```python
from build123d import *

# Parameters (mm, degrees)
F0_R     = 2
F0_R_2   = 2.2544770367
F1_DEPTH = 2


# Not quite as in the source:
# - ends of sketch curves that miss each other by under 0.0002 mm in the source are joined


with BuildPart() as f1:
    # F0 (on Top) → F1 (new body)
    with BuildSketch(Plane.XY):
        with BuildLine():
            ThreePointArc((-5.1683257468, -1.8810659147), (0, -5.5), (5.1683257468, -1.8810659147))
            Line((5.1683257468, -1.8810659147), (8.0301481547, -37.2918741238))
            ThreePointArc((8.0301481547, -37.2918741238), (9.2788304803, -38.3188106152), (10.2640215975, -37.0369352038))
            Line((10.2640215975, -37.0369352038), (3.1098692343, 51.4850906656))
            ThreePointArc((3.1098692343, 51.4850906656), (3.2758505583, 55.7142948477), (4.0791085727, 59.8698326439))
            Line((4.0791085727, 59.8698326439), (4.6310273864, 62.2435739623))
            ThreePointArc((4.6310273864, 62.2435739623), (6.6977396132, 71.4003991777), (3.5793046773, 80.2544440729))
            ThreePointArc((3.5793046773, 80.2544440729), (2.9779070013, 81.3790562482), (2.6805769718, 82.6192282376))
            Line((2.6805769718, 82.6192282376), (2.0130627379, 88.8089160456))
            ThreePointArc((2.0130627379, 88.8089160456), (1.9844093078, 88.9043745509), (1.9233044553, 88.9831117232))
            Line((1.9233044553, 88.9831117232), (0.9, 89.8927152157))
            Line((0.9, 89.8927152157), (0.9, 77.4665676321))
            ThreePointArc((0.9, 77.4665676321), (3.1034376701, 73.0014155649), (2.7328648238, 68.0359955106))
            ThreePointArc((2.7328648238, 68.0359955106), (1.8069828059, 67.0668885057), (0.5256445201, 66.6736988627))
            ThreePointArc((0.5256445201, 66.6736988627), (0.2620789214, 66.6755874914), (0, 66.7036058899))
            ThreePointArc((0, 66.7036058899), (-0.2620789214, 66.6755874914), (-0.5256445201, 66.6736988627))
            ThreePointArc((-0.5256445201, 66.6736988627), (-1.8069828059, 67.0668885057), (-2.7328648238, 68.0359955106))
            ThreePointArc((-2.7328648238, 68.0359955106), (-3.1034376701, 73.0014155649), (-0.9, 77.4665676321))
            Line((-0.9, 77.4665676321), (-0.9, 89.8927152157))
            Line((-0.9, 89.8927152157), (-1.9233044553, 88.9831117232))
            ThreePointArc((-1.9233044553, 88.9831117232), (-1.9844093078, 88.9043745509), (-2.0130627379, 88.8089160456))
            Line((-2.0130627379, 88.8089160456), (-2.6805769718, 82.6192282376))
            ThreePointArc((-2.6805769718, 82.6192282376), (-2.9779070013, 81.3790562482), (-3.5793046773, 80.2544440729))
            ThreePointArc((-3.5793046773, 80.2544440729), (-6.6977396132, 71.4003991777), (-4.6310273864, 62.2435739623))
            Line((-4.6310273864, 62.2435739623), (-4.0791085727, 59.8698326439))
            ThreePointArc((-4.0791085727, 59.8698326439), (-3.2758505583, 55.7142948477), (-3.1098692343, 51.4850906656))
            Line((-3.1098692343, 51.4850906656), (-10.2640215975, -37.0369352038))
            Line((-10.2640215975, -37.0369352038), (-10.264126962, -37.0382389339))
            ThreePointArc((-10.264126962, -37.0382389339), (-9.2781820506, -38.3188844261), (-8.0301481547, -37.2918741238))
            Line((-8.0301481547, -37.2918741238), (-5.1683257468, -1.8810659147))
        make_face()
        Circle(F0_R, mode=Mode.SUBTRACT)
        with BuildLine():
            ThreePointArc((4.7991758084, 2.6866171219), (0, 5.5), (-4.7991758084, 2.6866171219))
            Line((-4.7991758084, 2.6866171219), (-0.3733170252, 57.4500560059))
            ThreePointArc((-0.3733170252, 57.4500560059), (0, 57.4349952343), (0.3733170252, 57.4500560059))
            Line((0.3733170252, 57.4500560059), (4.7991758084, 2.6866171219))
        make_face(mode=Mode.SUBTRACT)
        with Locations((0, 62.0693005621)):
            Circle(F0_R_2, mode=Mode.SUBTRACT)
    extrude(amount=F1_DEPTH)


solid = f1.part
```
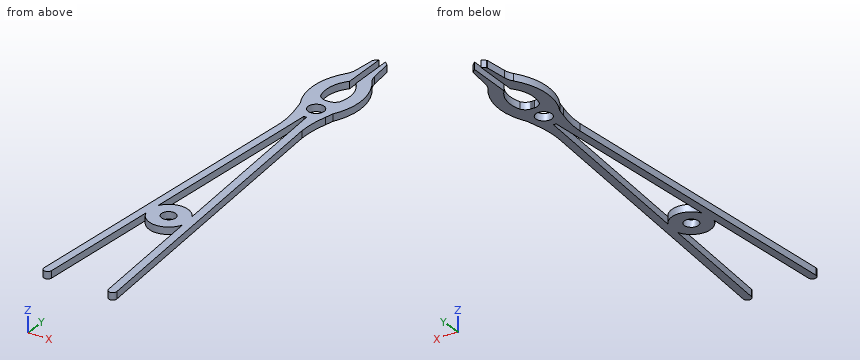
Can you work these out from the model? Positions are in its coordinate system, mm. Round coordinates to 2 decimals unless told otherwise and drop trailing zeros. Loops run counter-clockwise (first coordinate to the right, second up) from the corner with the lowest first, then second, coordinate; pieces in that order, holes last. Notation, with made-up numbers: M 87,-17.75 L 97,-17.75 A30 ccw 97,20.25 Z; hole C -9.75,-24 d8. An arc over 180 degrees is marked long. Answer as a JSON object with one key per item and string values. Group by question number.
Q1. Imagine slicing it at C-C, the plane z = 1.3. Count the separate pieces of the cut face and the enclosed holes in it, then the cut area to 3 significant figures.
Q2. Will this pin go through, and if not, where does the flat tip stop? pin 1 (1 mm diameter, centred on y = -15, z = 0.5, fed in from +X).
Q3. Imagine slicing it at A-A, the plane y = 0. Please give me the cut outline in (x, z), then the cut area to 3 significant figures.
Q4. Imagine slicing it at B-B, the plane y = 26. Please give me the cut outline in (x, z), then the cut area to 3 significant figures.
Q5. Please list where these lines run through material, in increasing order: L1, parallel to X at y = 61, z = 0.55; L2, parallel to X at y = 25, z = 0.6.
Findings:
{
 "1": {"separate pieces": "1", "enclosed holes": "3", "area": "716 mm2"},
 "2": {"pin 1": "stops at x = 8.52"},
 "3": {"outline": "M -7.27,0 L -2,0 L -2,2 L -7.27,2 Z; M 2,0 L 7.27,0 L 7.27,2 L 2,2 Z", "area": "21.1 mm2"},
 "4": {"outline": "M -5.17,0 L -2.92,0 L -2.92,2 L -5.17,2 Z; M 2.92,0 L 5.17,0 L 5.17,2 L 2.92,2 Z", "area": "9.02 mm2"},
 "5": {"L1": "x = -4.34 to -1.98, 1.98 to 4.34", "L2": "x = -5.25 to -3, 3 to 5.25"}
}
